Autodesk Inventor part; units mm, degrees
ref_plane "YZ Plane" through (0, 0, 0) normal (1, 0, 0) x (0, 1, 0)
ref_plane "XZ Plane" through (0, 0, 0) normal (0, 1, 0) x (-1, 0, 0)
ref_plane "XY Plane" through (0, 0, 0) normal (0, 0, 1) x (1, 0, 0)
sketch "Sketch1" plane through (0, 0, 0) normal (0, 1, 0) x (-1, 0, 0)
  line L0 (-15, 10) -> (20.359, 10)
  line L1 (25, 7.3205) -> (15, -10) construction
  line L2 (15, -10) -> (-15, -10)
  line L3 (-15, -10) -> (-15, 10)
  line L4 (-15, 10) -> (15, -10) construction
  line L5 (15, 10) -> (-15, -10) construction
  line L6 (20.359, 10) -> (55.6218, -10.359)
  line L7 (58.3013, -15) -> (40.9808, -25) construction
  line L8 (40.9808, -25) -> (15, -10)
  line L9 (15, -10) -> (15, 10) construction
  line L10 (55.6218, -10.359) -> (73.3013, -40.9808)
  line L11 (73.3013, -40.9808) -> (55.9808, -50.9808)
  line L12 (55.9808, -50.9808) -> (40.9808, -25)
  line L13 (40.9808, -25) -> (50.9808, -7.6795) construction
  point P0 (0, 0)
  point P1 (15, -10)
  dimension "d0" = 30
extrude "Extrusion1" add sketch "Sketch1" along normal blind 20
shell "Shell1" thickness 2 removed faces 2 at (-61.7543, 6.6667, -47.6474) at (15, 6.6667, 3.3333)
properties part number "finger_two_bend_hollow"
Read the model definition and answer for the solid it produces. Units are mm, in the model's axes. A direction names the side the tool comes from. Give positions to 0.01 mm unless a question says otherwise; leave off trailing zeros. Loops run counter-clockwise (first coordinate to the right, second up) from the corner with the lowest first, then second, coordinate; pieces in that order, holes last.
Item 1: The part is cut by section B-B (y = 10.5). Write down the section's boundary in (x, z).
Item 2: Each of these flat-tipped pins is pushed along its axis until it touches: pin 1 Ø5 at (y, z) = (6.5, -32.5) entering from +X; pin 2 Ø3 at (x, y) = (-53, 4.5) entering from -Z; pin 3 Ø2 at (y, z) = (7.5, -6.5) entering from +X. Where does it stop, or does it pass through?
Item 3: The part is cut by section C-C (z = -16.5). Write down the section's boundary in (x, y).
Item 4: Find the intervals of material crossed by line 1 along Y through (x, z) = (7, 3.5); line 2 along Z through (x, y) = (-11.5, 11.5); line 3 along Z through (x, y) = (-35, 4), in increasing order.
Item 5: The mould has two halves that part along X. Classify faces 1 (the flat face through (15, 19, 0)), 2 (the flat face through (0, 10, -8)), 3 (the flat face through (-29.179, 9.888, -15.877)): released by +X, released by -X, zero draft, split by the parting line, or undercut.
Item 6: The part is cut by section D-D (z = -3). Write down the section's boundary in (x, y), and give its area (3 significant figures).
Item 7: For faces 4 (the flat face through (-2, 10, 8)), 5 (the flat face through (0, 10, -10)), 6 (the flat face through (-50.186, 9.888, -36.943)), determine the directions among +Z, -Z, +X, -X, +Y, -Y from which every point of the face is accessible in a straight line to the end or side of a thin tool.
Item 8: The part is cut by section A-A (x = 4.5). Write down the section's boundary in (y, z), and give its area (3 significant figures).
Taken from the geometry:
1. outline: (-73.3, -40.98) - (-71.57, -41.98) - (-54.16, -11.82) - (-19.82, 8) - (15, 8) - (15, 10) - (-20.36, 10) - (-55.62, -10.36) - close; (-57.71, -49.98) - (-55.98, -50.98) - (-40.98, -25) - (-15, -10) - (15, -10) - (15, -8) - (-15.54, -8) - (-42.44, -23.54) - close
2. pin 1: stops at x = -43.87
2. pin 2: stops at z = -48.42
2. pin 3: stops at x = -43.21
3. outline: (-59.17, 0) - (-26.26, 0) - (-26.26, 20) - (-59.17, 20) - close; hole (-56.86, 2) - (-30.26, 2) - (-30.26, 18) - (-56.86, 18) - close
4. line 1: y = 0 to 2, 18 to 20
4. line 2: z = -10 to -8, 8 to 10
4. line 3: z = -21.55 to -19.24, -0.76 to 1.55
5. face 1: released by +X
5. face 2: zero draft
5. face 3: undercut
6. outline: (-42.88, 0) - (15, 0) - (15, 2) - (-38.88, 2) - (-38.88, 18) - (15, 18) - (15, 20) - (-42.88, 20) - close
6. area: 296 mm2
7. face 4: +X
7. face 5: -Z, +X, +Y, -Y
7. face 6: none
8. outline: (0, -10) - (20, -10) - (20, 10) - (0, 10) - close; hole (2, -8) - (18, -8) - (18, 8) - (2, 8) - close
8. area: 144 mm2
